Source: CAD feature listing. Evaluate the final solid. Frame: model axes, mm. Face numbers are marked on the shaded views. A direction names the side the tool comes from. Give positions to 0.01 mm unless a question says otherwise; leave off trailing zeros. Order: outer loops, then holes, each group sorted by start corner. A loop starts at its lowest first (then second) coordinate and runs counter-clockwise, first axis right, second up. Notation, with made-up numbers: (17, -25.5) - (43, -25.5) arc R23 cw to (43, -9.5) - close; hole circle Ø2 at (76.5, 3.5). An arc over 180 degrees is marked (long way). Use CSV: the item, a comma, the result in double quotes.
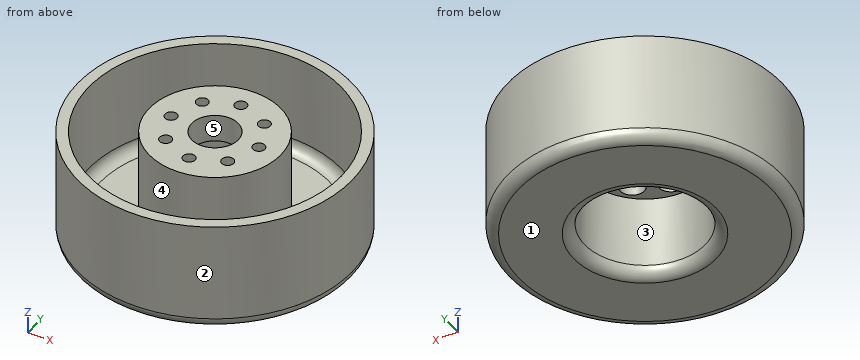
```python
from build123d import *

# Parameters (mm, degrees)
SKETCH1_R                      = 25
BOSS_EXTRUDE1_DEPTH            = 20
SKETCH4_R                      = 11
CUT_EXTRUDE1_DEPTH             = 15
CBORE_FOR_M2_SHCS2_D           = 2.2
CBORE_FOR_M2_SHCS2_CBORE_D     = 4.4
CBORE_FOR_M2_SHCS2_CBORE_DEPTH = 2
SKETCH7_R                      = 23
SKETCH7_R_2                    = 12
CUT_EXTRUDE2_DEPTH             = 18
FILLET1_R                      = 2
SKETCH8_R                      = 4.25
CUT_EXTRUDE3_DEPTH             = 18


with BuildPart() as part:
    # Sketch1 → Boss-Extrude1 (new body)
    with BuildSketch(Plane.XY):
        Circle(SKETCH1_R)
    extrude(amount=BOSS_EXTRUDE1_DEPTH)

    # Sketch4 → Cut-Extrude1 (cut)
    with BuildSketch(Plane(origin=(0, 0, 0), x_dir=(-1, 0, 0), z_dir=(0, 0, -1))):
        Circle(SKETCH4_R)
    extrude(amount=-CUT_EXTRUDE1_DEPTH, mode=Mode.SUBTRACT)

    # CBORE for M2 SHCS2 (through all)
    with Locations(Plane(origin=(0, 0, 15), x_dir=(-1, 0, 0), z_dir=(0, 0, -1))):
        with Locations((0, 8), (5.656854249, 5.656854249), (8, 0), (5.656854249, -5.656854249), (0, -8), (-5.656854249, -5.656854249), (-8, 0), (-5.656854249, 5.656854249)):
            CounterBoreHole(CBORE_FOR_M2_SHCS2_D / 2, CBORE_FOR_M2_SHCS2_CBORE_D / 2, CBORE_FOR_M2_SHCS2_CBORE_DEPTH)

    # Sketch7 → Cut-Extrude2 (cut)
    with BuildSketch(Plane.XY.offset(20)):
        Circle(SKETCH7_R)
        Circle(SKETCH7_R_2, mode=Mode.SUBTRACT)
    extrude(amount=-CUT_EXTRUDE2_DEPTH, mode=Mode.SUBTRACT)

    # Fillet1
    fillet1_edges = [part.edges().sort_by_distance(p)[0] for p in [
        (-25, 0, 0),
        (11, 0, 0),
        (-23, 0, 2),
    ]]
    fillet(fillet1_edges, radius=FILLET1_R)

    # Sketch8 → Cut-Extrude3 (cut)
    with BuildSketch(Plane.XY.offset(20)):
        Circle(SKETCH8_R)
    extrude(amount=-CUT_EXTRUDE3_DEPTH, mode=Mode.SUBTRACT)


solid = part.part
```
Item 1: Section A-A on z = 13.25. Return the cut outline in (x, y), then the cut area to 3 significant figures.
Filled in:
outline,"circle Ø50 at (0, 0); circle Ø24 at (0, 0); hole circle Ø46 at (0, 0); hole circle Ø22 at (0, 0)"
area,"374 mm2"
Item 2: Section B-B on y = 0. Count the separate pieces of the cut face and the enclosed holes in it, then the cut area to 3 significant figures.
Filled in:
separate pieces,"4"
enclosed holes,"0"
area,"199 mm2"
Item 3: Material intervals for line 1 (Y direction, x = 0, z = 16.25); line 2 (Y direction, x = 0, z = 18.05); line 3 (X direction, y = 1, z = 12.75), sorted ascending. Write a range as from..to.
Filled in:
line 1,"y = -25..-23, -12..-10.2, -5.8..-4.25, 4.25..5.8, 10.2..12, 23..25"
line 2,"y = -25..-23, -12..-9.1, -6.9..-4.25, 4.25..6.9, 9.1..12, 23..25"
line 3,"x = -24.98..-22.98, -11.96..-10.95, 10.95..11.96, 22.98..24.98"
Item 4: First-contact query: pin 1 (12 mm diameter, centred on y = -19, z = 8, fed in from +X); pin 2 (5 mm diameter, centred on y = -12, z = 7, fed in from -X); pin 3 (8 mm diameter, centred on y = 7, z = 7, fed in from -X). Flat tips, straight axial feed; report the tip coordinate or a pass-through.
Filled in:
pin 1,"stops at x = 21.35"
pin 2,"stops at x = -23.12"
pin 3,"stops at x = -24.82"
Item 5: Mould query, pull axis Y, two halves, no side actions, for the marked faces 1, 2 and 3. Classes: released by +Y, released by -Y, zero draft, split by the parting line, or undercut.
Filled in:
face 1,"zero draft"
face 2,"split by the parting line"
face 3,"undercut"
Item 6: Set-up query: the marked faces 4 and 5. Return all of +Z, -Z, +X, -X, +Y, -Y with unobstructed straight access to the full face (end or side cutting, diameter ignored); none if empty.
Filled in:
face 4,"+Z"
face 5,"+Z, -Z"
